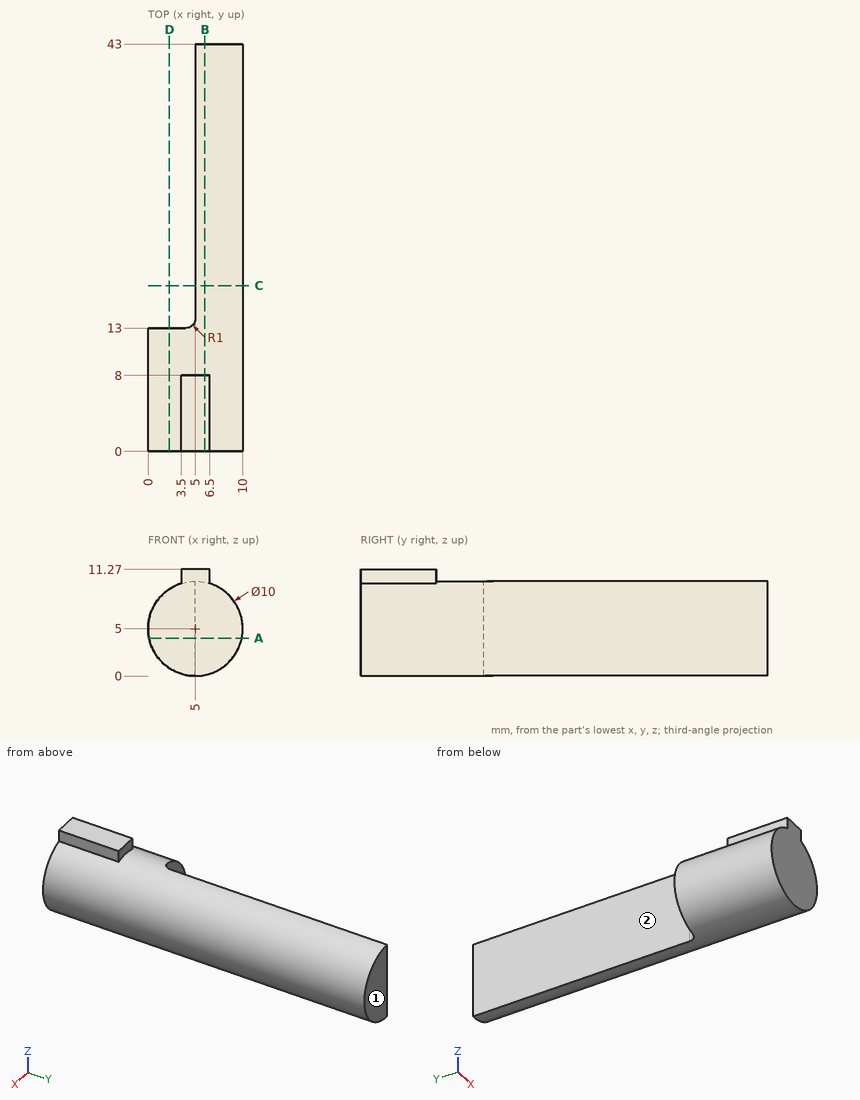
For this review, use the dimensioned drawing (mm, ordinates from the lowest corner) and the shaded views. A direction names the side the tool comes from. Round coordinates to 2 decimals unless told otherwise and drop trailing zeros. Write each loop counter-clockwise with the first axis right and the second up, starting at its lowest first coordinate (ties: lowest second). Pieces come first, ordered by that corner, then holes. Notation, with made-up numbers: (5.5, -12) - (30.5, -12) arc R22 cw to (30.5, 12) - close; hole circle Ø9 at (-3, 43). An arc over 180 degrees is marked (long way). Use a Markdown table: item, result.
Q1. We need section A-A (z = 4). Give the boundary of the cut face in (x, y).
Derived:
| item | result |
|---|---|
| outline | (0.1, 0) - (9.9, 0) - (9.9, 43) - (5, 43) - (5, 14) arc R1 cw to (4, 13) - (0.1, 13) - close |
Q2. We need section D-D (x = 2.25). Give the boundary of the cut face in (y, z).
Derived:
| item | result |
|---|---|
| outline | (0, 0.82) - (13, 0.82) - (13, 9.18) - (0, 9.18) - close |
Q3. Clearance check with flat-ended pins moving along their axes: pin 1 (0.8 mm diameter, centred on y = 4.5, z = 10.5, fed in from -X); pin 2 (1 mm diameter, centred on y = 7, z = 7.5, fed in from +X); pin 3 (4.5 mm diameter, centred on x = 1, z = 6.5, fed in from +Y). State where each tip first meets the part, or that it passes through.
Derived:
| item | result |
|---|---|
| pin 1 | stops at x = 3.5 |
| pin 2 | stops at x = 9.58 |
| pin 3 | stops at y = 13 |
Q4. Wall thickness on line 1 along X through (y, z) = (27.5, 9); line 2 along Y through (x, z) = (1.75, 3.5); line 3 along X through (y, z) = (4, 4): over which ranges is each line inside the solid? List them lowest first.
Derived:
| item | result |
|---|---|
| line 1 | x = 5 to 8 |
| line 2 | y = 0 to 13 |
| line 3 | x = 0.1 to 9.9 |
Q5. Machinability: for the marked faces 1 and 2, which of the approach directions +Z, -Z, +X, -X, +Y, -Y give a long, thin tool a straight path to every point of the face, cutting with its end or side? Answer none if there is none.
Derived:
| item | result |
|---|---|
| face 1 | +Z, -Z, +X, -X, +Y |
| face 2 | +Z, -Z, -X, +Y |
Q6. We need section C-C (y = 17.5). Give the boundary of the cut face in (x, z), plus the area to 3 significant figures.
Derived:
| item | result |
|---|---|
| outline | (5, 0) arc R5 ccw to (5, 10) - close |
| area | 39.3 mm2 |
Q7. We need section B-B (x = 6). Give the boundary of the cut face in (y, z).
Derived:
| item | result |
|---|---|
| outline | (0, 0.1) - (43, 0.1) - (43, 9.9) - (8, 9.9) - (8, 11.27) - (0, 11.27) - close |
